Verification items for the finished model (mm, model axes). A direction names the side the tool comes from. Round coordinates to 2 decimals unless told otherwise and drop trailing zeros. Loops run counter-clockwise (first coordinate to the right, second up) from the corner with the lowest first, then second, coordinate; pieces in that order, holes last.
from build123d import *

# Parameters (mm, degrees)
SKETCH1_W           = 1200
SKETCH1_H           = 2200
SKETCH1_W_2         = 1000
SKETCH1_H_2         = 2000
BOSS_EXTRUDE1_DEPTH = 100
SKETCH2_R           = 25
CUT_EXTRUDE1_DEPTH  = 2373.762103541


with BuildPart() as part:
    # Sketch1 → Boss-Extrude1 (new body)
    with BuildSketch(Plane.XY):
        with Locations((500, 1000)):
            Rectangle(SKETCH1_W, SKETCH1_H)
        with Locations((500, 1000)):
            Rectangle(SKETCH1_W_2, SKETCH1_H_2, mode=Mode.SUBTRACT)
    extrude(amount=BOSS_EXTRUDE1_DEPTH)

    # Sketch2 → Cut-Extrude1 (cut, through all)
    with BuildSketch(Plane.XY.offset(100)):
        with Locations((1050, 1900)):
            Circle(SKETCH2_R)
        with Locations((1050, 100)):
            Circle(SKETCH2_R)
    extrude(amount=-CUT_EXTRUDE1_DEPTH, mode=Mode.SUBTRACT)


solid = part.part
1. Release check for a two-part mould opening along Y. For faces 3 (the face through (-36, 1005, 100)), 4 (the face through (493, 0, 49)), 5 (the face through (492, -100, 49)) record: released by +Y, released by -Y, zero draft, split by the parting line, or undercut.
2. Section check D-D (z = 26.5). Enter the section's corners in (x, y), then the cut area to 3 significant figures.
3. Section check B-B (y = 100). Enter the section's corners in (x, z), then the cut area to 3 significant figures.
4. Section check A-A (x = 1050). Enter the section's corners in (y, z), then the cut area to 3 significant figures.
5. Section check C-C (y = 1450.5). Enter the section's corners in (x, z).
6. Scan lines: L1, parallel to Y at x = 1050, z = 49; L2, parallel to X at y = 1900, z = 31; L3, parallel to X at y = 401.5, z = 20.5. Record each from-to range of solid material in increasing order.
7. Tool access check on faces 1 (the face through (1000, 986, 49)), 2 (the face through (1100, 985, 49)). Record the directions out of +Z, -Z, +X, -X, +Y, -Y that give a thin tool (end or side, any length) a straight path to the whole face; none if there is none.
Taken from the geometry:
1. face 3: zero draft
1. face 4: undercut
1. face 5: released by -Y
2. outline: (-100, -100) - (1100, -100) - (1100, 2100) - (-100, 2100) - close; hole (0, 0) - (1000, 0) - (1000, 2000) - (0, 2000) - close; hole circle Ø50 at (1050, 100); hole circle Ø50 at (1050, 1900)
2. area: 636,000 mm2
3. outline: (-100, 0) - (0, 0) - (0, 100) - (-100, 100) - close; (1000, 0) - (1025, 0) - (1025, 100) - (1000, 100) - close; (1075, 0) - (1100, 0) - (1100, 100) - (1075, 100) - close
3. area: 15,000 mm2
4. outline: (-100, 0) - (75, 0) - (75, 100) - (-100, 100) - close; (125, 0) - (1875, 0) - (1875, 100) - (125, 100) - close; (1925, 0) - (2100, 0) - (2100, 100) - (1925, 100) - close
4. area: 210,000 mm2
5. outline: (-100, 0) - (0, 0) - (0, 100) - (-100, 100) - close; (1000, 0) - (1100, 0) - (1100, 100) - (1000, 100) - close
6. L1: y = -100 to 75, 125 to 1875, 1925 to 2100
6. L2: x = -100 to 0, 1000 to 1025, 1075 to 1100
6. L3: x = -100 to 0, 1000 to 1100
7. face 1: +Z, -Z
7. face 2: +Z, -Z, +X, +Y, -Y
